Source: CAD feature listing. Evaluate the final solid. Frame: model axes, mm. A direction names the side the tool comes from. Round coordinates to 2 decimals unless told otherwise and drop trailing zeros. Write each loop counter-clockwise with the first axis right and the second up, starting at its lowest first coordinate (ties: lowest second). Pieces come first, ordered by that corner, then holes. Notation, with made-up numbers: (-11, 11.25) -> (35, 11.25) arc R35 ccw to (35, 46.25) -> close; hole circle Ø8 at (-7, 22). An arc over 180 degrees is marked (long way). Return JSON: item names as keys, results as strings. Group by question number.
from build123d import *

# Parameters (mm, degrees)
CROQUIS3_W              = 110.308657866
CROQUIS3_H              = 110.308657866
CROQUIS3_R              = 1.25
CROQUIS3_R_2            = 3
SALIENTE_EXTRUIR1_DEPTH = 3


with BuildPart() as part:
    # Croquis3 → Saliente-Extruir1 (new body)
    with BuildSketch(Plane.XY):
        Rectangle(CROQUIS3_W, CROQUIS3_H)
        with Locations((-8.838834765, 8.838834765)):
            Circle(CROQUIS3_R, mode=Mode.SUBTRACT)
        with Locations((8.838834765, 8.838834765)):
            Circle(CROQUIS3_R, mode=Mode.SUBTRACT)
        with Locations((8.838834765, -8.838834765)):
            Circle(CROQUIS3_R, mode=Mode.SUBTRACT)
        with Locations((-8.838834765, -8.838834765)):
            Circle(CROQUIS3_R, mode=Mode.SUBTRACT)
        with Locations((-49.497474683, 49.497474683)):
            Circle(CROQUIS3_R_2, mode=Mode.SUBTRACT)
        with Locations((49.497474683, 49.497474683)):
            Circle(CROQUIS3_R_2, mode=Mode.SUBTRACT)
        with Locations((49.497474683, -49.497474683)):
            Circle(CROQUIS3_R_2, mode=Mode.SUBTRACT)
        with Locations((-49.497474683, -49.497474683)):
            Circle(CROQUIS3_R_2, mode=Mode.SUBTRACT)
        with BuildLine():
            Line((25, -10), (25, 10))
            ThreePointArc((25, 10), (32.5, 17.5), (40, 10))
            Line((40, 10), (40, -10))
            ThreePointArc((40, -10), (32.5, -17.5), (25, -10))
        make_face(mode=Mode.SUBTRACT)
        with BuildLine():
            Line((-25, -10), (-25, 10))
            ThreePointArc((-25, 10), (-32.5, 17.5), (-40, 10))
            Line((-40, 10), (-40, -10))
            ThreePointArc((-40, -10), (-32.5, -17.5), (-25, -10))
        make_face(mode=Mode.SUBTRACT)
        with BuildLine():
            Line((-10, 40), (10, 40))
            ThreePointArc((10, 40), (17.5, 32.5), (10, 25))
            Line((10, 25), (-10, 25))
            ThreePointArc((-10, 25), (-17.5, 32.5), (-10, 40))
        make_face(mode=Mode.SUBTRACT)
        with BuildLine():
            Line((-10, -40), (10, -40))
            ThreePointArc((10, -40), (17.5, -32.5), (10, -25))
            Line((10, -25), (-10, -25))
            ThreePointArc((-10, -25), (-17.5, -32.5), (-10, -40))
        make_face(mode=Mode.SUBTRACT)
    extrude(amount=SALIENTE_EXTRUIR1_DEPTH)


solid = part.part
Item 1: Cut plane C-C on x = -32.5. Output: boundary loops of the cut face in (y, z).
Item 2: Material intervals for probe 1 along X at (y, z) = (-1.5, 0.55); probe 2 along Y at (x, z) = (11, 2.15), sorted ascending.
Item 3: Set-up query: faces 4 (the flat face through (0, -40, 1)), 5 (the flat face through (-1, -55.154, 1)). Return all of +Z, -Z, +X, -X, +Y, -Y with unobstructed straight access to the full face (end or side cutting, diameter ignored); none if empty.
Item 4: Pull-direction query (Y, two-part tool) for faces 1 (the flat face through (-1, 55.154, 1)), 2 (the cylindrical face through (46.5, -49.4, 1.5)), 3 (the flat face through (-1, 1, 3)); classes: +Y half, -Y half, draft (parallel to the pull), parting line (faces both ways), or undercut.
Item 5: First-contact query: pin 1 Ø1.5 at (x, y) = (-8.84, 8.84) entering from +Z. Flat tip, straight axial feed; report the tip coordinate or a pass-through.
Item 6: Cut plane A-A on y = -6. Output: boundary loops of the cut face in (x, z), and give its area (3 significant figures).
Here are the results:
{
 "1": {"outline": "(-55.15, 0) -> (-17.5, 0) -> (-17.5, 3) -> (-55.15, 3) -> close; (17.5, 0) -> (55.15, 0) -> (55.15, 3) -> (17.5, 3) -> close"},
 "2": {"probe 1": "x = -55.15 to -40, -25 to 25, 40 to 55.15", "probe 2": "y = -55.15 to -39.93, -25.07 to 25.07, 39.93 to 55.15"},
 "3": {"face 4": "+Z, -Z", "face 5": "+Z, -Z, +X, -X, -Y"},
 "4": {"face 1": "+Y half", "face 2": "undercut", "face 3": "draft"},
 "5": {"pin 1": "passes through"},
 "6": {"outline": "(-55.15, 0) -> (-40, 0) -> (-40, 3) -> (-55.15, 3) -> close; (-25, 0) -> (25, 0) -> (25, 3) -> (-25, 3) -> close; (40, 0) -> (55.15, 0) -> (55.15, 3) -> (40, 3) -> close", "area": "241 mm^2"}
}
